from build123d import *

# Parameters (mm, degrees)
F1_DEPTH = 25.2984


with BuildPart() as f1:
    # F0 (on Front) → F1 (new body)
    with BuildSketch(Plane.XZ):
        with BuildLine():
            ThreePointArc((76.2, -30.48), (45.72, 0), (76.2, 30.48))
            Line((76.2, 30.48), (-76.2, 30.48))
            ThreePointArc((-76.2, 30.48), (-54.6473853094, 21.5526146906), (-45.72, 0))
            ThreePointArc((-45.72, 0), (-54.6473853094, -21.5526146906), (-76.2, -30.48))
            Line((-76.2, -30.48), (76.2, -30.48))
        make_face()
        with BuildLine():
            ThreePointArc((106.68, 0), (97.7526146906, 21.5526146906), (76.2, 30.48))
            Line((76.2, 30.48), (76.2, 19.05))
            ThreePointArc((76.2, 19.05), (89.6703841816, 13.4703841816), (95.25, 0))
            ThreePointArc((95.25, 0), (89.6703841816, -13.4703841816), (76.2, -19.05))
            Line((76.2, -19.05), (76.2, -30.48))
            ThreePointArc((76.2, -30.48), (97.7526146906, -21.5526146906), (106.68, 0))
        make_face()
        with BuildLine():
            Line((76.2, 19.05), (76.2, 30.48))
            ThreePointArc((76.2, 30.48), (45.72, 0), (76.2, -30.48))
            Line((76.2, -30.48), (76.2, -19.05))
            ThreePointArc((76.2, -19.05), (57.15, 0), (76.2, 19.05))
        make_face()
        with BuildLine():
            ThreePointArc((-45.72, 0), (-54.6473853094, 21.5526146906), (-76.2, 30.48))
            Line((-76.2, 30.48), (-76.2, 19.05))
            ThreePointArc((-76.2, 19.05), (-62.7296158184, 13.4703841816), (-57.15, 0))
            ThreePointArc((-57.15, 0), (-62.7296158184, -13.4703841816), (-76.2, -19.05))
            Line((-76.2, -19.05), (-76.2, -30.48))
            ThreePointArc((-76.2, -30.48), (-54.6473853094, -21.5526146906), (-45.72, 0))
        make_face()
        with BuildLine():
            Line((-76.2, 19.05), (-76.2, 30.48))
            ThreePointArc((-76.2, 30.48), (-106.68, 0), (-76.2, -30.48))
            Line((-76.2, -30.48), (-76.2, -19.05))
            ThreePointArc((-76.2, -19.05), (-95.25, 0), (-76.2, 19.05))
        make_face()
    extrude(amount=F1_DEPTH)


solid = f1.part
The model under review builds one solid part; all positions refer to its coordinate system, in mm. Round coordinates to 2 decimals unless told otherwise and drop trailing zeros. Loops run counter-clockwise (first coordinate to the right, second up) from the corner with the lowest first, then second, coordinate; pieces in that order, holes last. Notation, with made-up numbers: (73, 74.5) - (131, 74.5) arc R20 cw to (131, 80.5) - close; hole circle Ø10 at (17.5, -14.75). An arc over 180 degrees is marked (long way). Use CSV: the item, a comma, the result in double quotes.
(1) Take a section at A-A, the plane y = -17. Give the boundary of the cut face in (x, z).
Working result:
outline,"(-76.2, -30.48) - (76.2, -30.48) arc R30.48 ccw to (76.2, 30.48) - (-76.2, 30.48) arc R30.48 ccw to start; hole circle Ø38.1 at (-76.2, 0); hole circle Ø38.1 at (76.2, 0)"
(2) The part is to be moulded in two halves that separate along Z. For faces 1 (the flat face through (1, -12, 30.48)), 2 (the cylindrical face through (72.07, -12.472, 18.597)), 3 (the cylindrical face through (-95.23, -12.47, -0.84)), 4 (the flat face through (-1, -25.298, 0)), say which applies: pulls with the +Z half, pulls with the -Z half, needs draft (parallel to the pull), parting line crosses it, or undercut.
Working result:
face 1,"pulls with the +Z half"
face 2,"undercut"
face 3,"undercut"
face 4,"needs draft"
(3) Take a section at B-B, the plane z = 4. Give the boundary of the cut face in (x, y), plus the area to 3 significant figures.
Working result:
outline,"(-106.42, -25.3) - (-94.83, -25.3) - (-94.83, 0) - (-106.42, 0) - close; (-57.57, -25.3) - (57.57, -25.3) - (57.57, 0) - (-57.57, 0) - close; (94.83, -25.3) - (106.42, -25.3) - (106.42, 0) - (94.83, 0) - close"
area,"3,500 mm^2"
(4) Take a section at C-C, the plane x = 80.5. Give the boundary of the cut face in (y, z), plus the area to 3 significant figures.
Working result:
outline,"(-25.3, -30.18) - (0, -30.18) - (0, -18.56) - (-25.3, -18.56) - close; (-25.3, 18.56) - (0, 18.56) - (0, 30.18) - (-25.3, 30.18) - close"
area,"588 mm^2"
(5) Take a section at D-D, the plane x = -81. Give the boundary of the cut face in (y, z), plus the area to 3 significant figures.
Working result:
outline,"(-25.3, -30.1) - (0, -30.1) - (0, -18.44) - (-25.3, -18.44) - close; (-25.3, 18.44) - (0, 18.44) - (0, 30.1) - (-25.3, 30.1) - close"
area,"590 mm^2"
(6) Clearance check with flat-ended pins moving along their axes: P1, Ø2, axis at y = -17, z = 12, coming from the -X side; P2, Ø8, axis at y = -20, z = -18.5, coming from the -X side. State where each tip first meets the part, or that it passes through.
Working result:
P1,"stops at x = -104.63"
P2,"stops at x = -103.01"
(7) For line 1 (X direction, y = -24, z = 1); line 2 (X direction, y = -16.5, z = 2); line 3 (Z direction, x = -76.2, y = -7.75), list the stretches that pass through material, from the lowest coordinate up.
Working result:
line 1,"x = -106.66 to -95.22, -57.18 to 57.18, 95.22 to 106.66"
line 2,"x = -106.61 to -95.14, -57.26 to 57.26, 95.14 to 106.61"
line 3,"z = -30.48 to -19.05, 19.05 to 30.48"
